Verification items for the finished model (mm, model axes). Round coordinates to 2 decimals unless told otherwise and drop trailing zeros. Write each loop counter-clockwise with the first axis right and the second up, starting at its lowest first coordinate (ties: lowest second). Pieces come first, ordered by that corner, then holes. Notation, with made-up numbers: M 19,-24 L 70,-24 A28 ccw 70,15 Z; hole C 38.25,19 d2. An arc over 180 degrees is marked long. Answer in a Markdown table with one row per item. Add a question column.
1. Draft check along X on faces 1 (the cylindrical face through (-5.806, 2.465, 3.735)), 2 (the flat face through (-5, 2, 10)), 3 (the flat face through (-10, 2, 5)). Enter one of: pulls with the +X half, pulls with the -X half, needs draft (parallel to the pull), parting line crosses it, or undercut.
2. Sectioned sample at A-A on y = 0.9. Record the cut outline in (x, z), plus the area to 3 significant figures.
3. Material ranges on probe 1 along Z at (x, y) = (-5, 2.7); probe 2 along X at (y, z) = (1.5, 4.75); probe 3 along X at (y, z) = (2.5, 4.5), recorded low to high.
4. Go/stop test with a flat-tipped pin: pin 1 Ø2 at (x, z) = (-5, 6) entering from -Y. Record where the tip stops, or that it passes through.
5. Sectioned sample at B-B on z = 5. Record the cut outline in (x, y).
6. Sectioned sample at C-C on x = -5. Record the cut outline in (y, z), plus the area to 3 significant figures.
Autodesk Inventor part; units mm, degrees
ref_plane "YZ Plane" through (0, 0, 0) normal (1, 0, 0) x (0, 1, 0)
ref_plane "XZ Plane" through (0, 0, 0) normal (0, 1, 0) x (-1, 0, 0)
ref_plane "XY Plane" through (0, 0, 0) normal (0, 0, 1) x (1, 0, 0)
sketch "Sketch1" plane through (0, 0, 0) normal (0, 1, 0) x (-1, 0, 0)
  line L0 (0, 0) -> (10, 0)
  line L1 (10, 0) -> (10, 10)
  line L2 (10, 10) -> (0, 10)
  line L3 (0, 10) -> (0, 0)
  circle A0 centre (5, 5) radius 1.5
  point P0 (10, 5)
  point P1 (5, 10)
  dimension "d0" = 10
  dimension "d1" = 10
  dimension "d4" = 3
extrude "Extrusion1" add sketch "Sketch1" along normal blind 5
properties part number "spacer"
Geometry check:
| question | item | result |
|---|---|---|
| 1 | face 1 | undercut |
| 1 | face 2 | needs draft |
| 1 | face 3 | pulls with the -X half |
| 2 | outline | M -10,0 L 0,0 L 0,10 L -10,10 Z; hole C -5,5 d3 |
| 2 | area | 92.9 mm2 |
| 3 | probe 1 | z = 0 to 3.5, 6.5 to 10 |
| 3 | probe 2 | x = -10 to -6.48, -3.52 to 0 |
| 3 | probe 3 | x = -10 to -6.41, -3.59 to 0 |
| 4 | pin 1 | stops at y = 0 |
| 5 | outline | M -10,0 L -6.5,0 L -6.5,5 L -10,5 Z; M -3.5,0 L 0,0 L 0,5 L -3.5,5 Z |
| 6 | outline | M 0,0 L 5,0 L 5,3.5 L 0,3.5 Z; M 0,6.5 L 5,6.5 L 5,10 L 0,10 Z |
| 6 | area | 35.0 mm2 |
